Study the drawing (mm; zero at the part's minimum x, y, z) and answer. A direction names the side the tool comes from. Coordinates: 2 decimals unless noted, no trailing zeros. Order: outer loops, then holes, each group sorted by start corner. A loop starts at its lowest first (then second) coordinate and runs counter-clockwise, first axis right, second up.
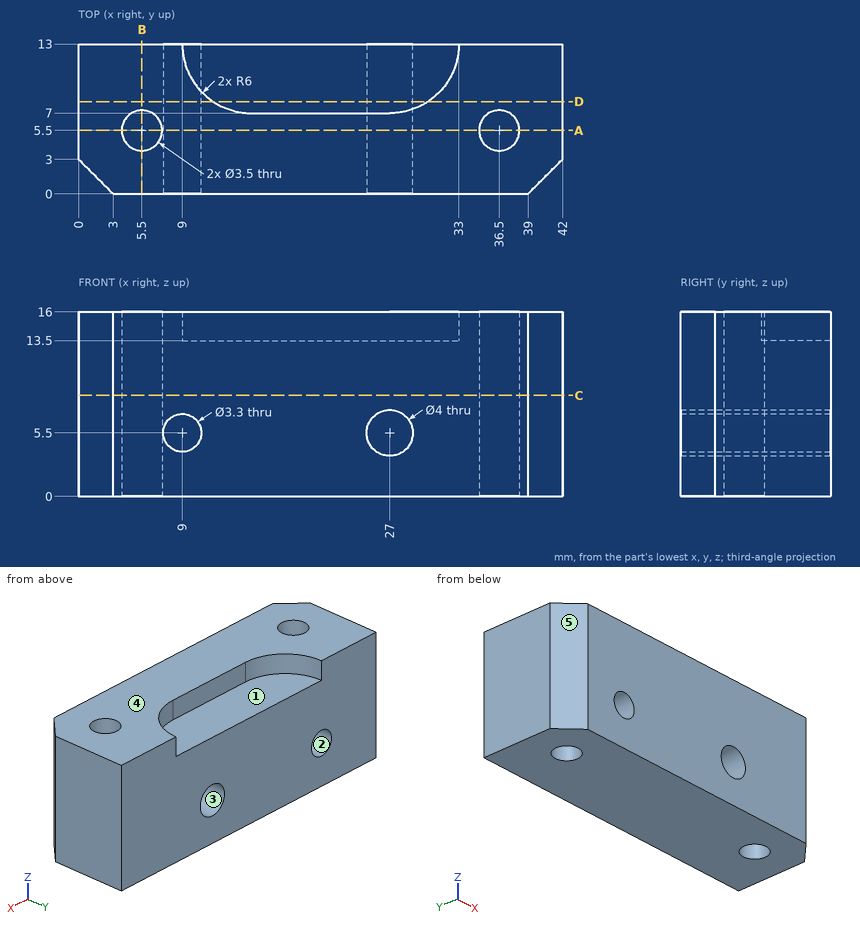
(1) The mould has two halves that part along X. Classify the marked faces 3, 4 and 5: pulls with the +X half, pulls with the -X half, needs draft (parallel to the pull), parting line crosses it, or undercut.
(2) Find section B-B on x = 5.5. Determine the outline of the cut face in (y, z), then the cut area to 3 significant figures.
(3) A tool of negligible diameter and unlimited length cuts with its end or side. For the marked faces 1 and 2, from which of +Z, -Z, +X, -X, +Y, -Y can it reach the whole face along a straight path? Write none if from no direction.
(4) Find section A-A on y = 5.5. Determine the outline of the cut face in (x, z), then the cut area to 3 significant figures.
(5) Find section C-C on z = 8.75. Determine the outline of the cut face in (x, y), then the cut area to 3 significant figures.
(6) Given pin 1 Ø6.5 at (x, y) = (25, 10.5) entering from +Z; pin 2 Ø3 at (x, z) = (9, 5.5) entering from -Y, each flat-ended and moving along its own axis, determine where each tip first touches the part or whether it passes through.
(7) Find the intervals of material crossed by probe 1 along Y at (x, z) = (5.5, 7.5); probe 2 along X at (y, z) = (4.25, 7); probe 3 along X at (y, z) = (6, 2.5), in increasing order.
(8) Find section D-D on y = 8. Determine the outline of the cut face in (x, z).
Resolved:
1. face 3: undercut
1. face 4: needs draft
1. face 5: pulls with the -X half
2. outline: (0, 0) - (3.75, 0) - (3.75, 16) - (0, 16) - close; (7.25, 0) - (13, 0) - (13, 16) - (7.25, 16) - close
2. area: 152 mm2
3. face 1: +Z, +Y
3. face 2: +Y, -Y
4. outline: (0, 0) - (3.75, 0) - (3.75, 16) - (0, 16) - close; (7.25, 0) - (34.75, 0) - (34.75, 16) - (7.25, 16) - close; (38.25, 0) - (42, 0) - (42, 16) - (38.25, 16) - close; hole circle Ø3.3 at (9, 5.5); hole circle Ø4 at (27, 5.5)
4. area: 539 mm2
5. outline: (0, 3) - (3, 0) - (39, 0) - (42, 3) - (42, 13) - (0, 13) - close; hole circle Ø3.5 at (5.5, 5.5); hole circle Ø3.5 at (36.5, 5.5)
5. area: 518 mm2
6. pin 1: stops at z = 13.5
6. pin 2: passes through
7. probe 1: y = 0 to 3.75, 7.25 to 13
7. probe 2: x = 0 to 4.28, 6.72 to 8.31, 9.69 to 25.68, 28.32 to 35.28, 37.72 to 42
7. probe 3: x = 0 to 3.82, 7.18 to 34.82, 38.18 to 42
8. outline: (0, 0) - (42, 0) - (42, 16) - (30.32, 16) - (30.32, 13.5) - (11.68, 13.5) - (11.68, 16) - (0, 16) - close; hole circle Ø3.3 at (9, 5.5); hole circle Ø4 at (27, 5.5)
